CAD build for the part. Positions are in the model's coordinates, mm. A direction names the side the tool comes from. Round coordinates to 2 decimals unless told otherwise and drop trailing zeros. Order: outer loops, then holes, each group sorted by start corner. A loop starts at its lowest first (then second) coordinate and runs counter-clockwise, first axis right, second up. Notation, with made-up numbers: M 57.5,-28 L 67.5,-28 A16 ccw 67.5,-4 Z; hole C 24.5,16.25 d11. An arc over 180 degrees is marked long. Answer as a JSON object with one key per item and string values.
Autodesk Inventor part; units mm, degrees
ref_plane "CNS_SCREW_XY" through (0, 0, 0) normal (0, 1, 0) x (1, 0, 0)
ref_plane "CNS_SCREW_YZ" through (0, 0, 0) normal (1, 0, 0) x (0, 0, -1)
ref_plane "CNS_SCREW_ZX" through (0, 0, 0) normal (0, 0, -1) x (0, 1, 0)
sketch "Sketch_1" plane through (0, 0, 0) normal (0, 0, 1) x (1, 0, 0)
  line L0 (0, -3.97) -> (0, 16.9)
  line L1 (0, 16.9) -> (4.85, 16.9)
  line L2 (4.85, 16.9) -> (4.85, 15.4)
  line L3 (4.85, 15.4) -> (3.4, 15.4)
  line L4 (3.4, 15.4) -> (3.4, 14.5)
  line L5 (3.4, 14.5) -> (5, 14.5)
  line L6 (5, 14.5) -> (5, 4)
  line L7 (5, 4) -> (4.9889, 4)
  line L8 (4.9889, 4) -> (4.7401, -3.97)
  line L9 (4.7401, -3.97) -> (0, -3.97)
  line L10 (0, -3.97) -> (0, 16.9)
revolve "Revolution1" add sketch "Sketch_1" angle 360 about axis through (0, -3.97, 0) along (0, -1, 0)
thread "Thread1"
sketch "_____1" plane through (0, 0, 0) normal (0, 0, 1) x (1, 0, 0)
  line L0 (-9.728, -3.1) -> (-9.728, -3.97)
  line L1 (-9.728, -3.97) -> (9.728, -3.97)
  line L2 (9.728, -3.97) -> (9.728, -3.1)
  line L3 (9.728, -3.1) -> (-9.728, -3.1)
extrude "Extrusion1" cut sketch "_____1" along normal mid plane 19.456
sketch "Sketch_2" plane through (0, 0, 0) normal (0, 0, 1) x (1, 0, 0)
  line L0 (0, 3.6) -> (0, 16.9)
  line L1 (0, 16.9) -> (3, 16.9)
  line L2 (3, 16.9) -> (3, 3.6)
  line L3 (3, 3.6) -> (0, 3.6)
  line L4 (0, 3.6) -> (0, 16.9)
revolve "Revolution2" cut sketch "Sketch_2" angle 360 about axis through (0, 3.6, 0) along (0, -1, 0)
sketch "Sketch_3" plane through (0, 16.9, 0) normal (0, 1, 0) x (1, 0, 0)
  line L0 (-2, -1.1547) -> (0, -2.3094)
  line L1 (0, -2.3094) -> (2, -1.1547)
  line L2 (2, -1.1547) -> (2, 1.1547)
  line L3 (2, 1.1547) -> (0, 2.3094)
  line L4 (0, 2.3094) -> (-2, 1.1547)
  line L5 (-2, 1.1547) -> (-2, -1.1547)
extrude "Extrusion2" cut sketch "Sketch_3" against normal blind 18.8
ref_plane "CNS_SCREW_XY" through (0, 0, 0) normal (0, 1, 0) x (1, 0, 0)
ref_plane "CNS_SCREW_YZ" through (0, 0, 0) normal (1, 0, 0) x (0, 0, -1)
ref_plane "CNS_SCREW_ZX" through (0, 0, 0) normal (0, 0, -1) x (0, 1, 0)
properties part number "KQ2S06-01AS (A) Brass"
Item 1: Wall check: line 1 along Z through (x, y) = (0, 11.5); line 2 along Y through (x, z) = (-2.5, -2.5); line 3 along Y through (x, z) = (1.5, 0.5). Give the ranges that are in metal, low to high. Write a range as [from, to].
Worked answers:
{"line 1": "z = [-5, -3], [3, 5]", "line 2": "y = [-3.1, 14.5], [15.4, 16.9]", "line 3": "y = [-3.1, -1.9]"}
Item 2: Two-plate mould, pull along X, no slides. Class faces 1 (the flat face through (-1, 3.6, -2)), 2 (the flat face through (3.2, 16.9, 0.1)), 3 (the cylindrical face through (-0.74, 14.94, -3.32)): released by +X, released by -X, zero draft, split by the parting line, or undercut.
Worked answers:
{"face 1": "undercut", "face 2": "zero draft", "face 3": "split by the parting line"}
Item 3: Drop flat-ended pins along their axis: pin 1 Ø0.7 at (y, z) = (2, 0.5) entering from +X; pin 2 Ø3 at (x, y) = (-1, -0.5) entering from -Z; pin 3 Ø1 at (y, z) = (4.5, -1) entering from +X. Give the stop position or say it passes through.
Worked answers:
{"pin 1": "stops at x = 4.93", "pin 2": "stops at z = -4.88", "pin 3": "stops at x = 4.97"}
Item 4: Saw through at B-B on y = 1.5. List the corners of the cut face in (x, z), and give its area (3 significant figures).
Worked answers:
{"outline": "C 0,0 d9.82; hole M -2,-1.15 L 0,-2.31 L 2,-1.15 L 2,1.15 L 0,2.31 L -2,1.15 Z", "area": "61.9 mm2"}
Item 5: Saw through at C-C on y = 9.75. List the corners of the cut face in (x, z).
Worked answers:
{"outline": "C 0,0 d10; hole C 0,0 d6"}
Item 6: 3-axis set-ups, long thin cutter, end or side, ignore diameter. For faces 4 (the conical face through (-1.058, 0.5, 4.764)), 5 (the flat face through (1.014, 0.889, -1.724)), 6 (the flat face through (3, 15.4, -2)), 7 (the cylindrical face through (-1.08, 9.18, -4.88)): which of +Z, -Z, +X, -X, +Y, -Y reach the whole face in a straight line?
Worked answers:
{"face 4": "-Y", "face 5": "+Y", "face 6": "none", "face 7": "+Y, -Y"}
